For this review, take the finished solid that the model builds, in its own axes (mm). Coordinates: 2 decimals unless noted, no trailing zeros. Loops run counter-clockwise (first coordinate to the right, second up) from the corner with the lowest first, then second, coordinate; pieces in that order, holes last. Notation, with made-up numbers: M -18.5,31 L -5.5,31 A15 ccw -5.5,42 Z; hole C 49.25,-35 d1. An arc over 180 degrees is marked long. Use one line per item in the form item = value.
```python
from build123d import *

# Parameters (mm, degrees)
BOSS_EXTRUDE1_START = 63.5
BOSS_EXTRUDE1_DEPTH = 12.7
CAVITY1_START       = 63.5
CAVITY1_OUTLINE_R   = 12.7
CAVITY1_DEPTH       = 12.7


# Read off the part's stored shape, not the designer's step: Cavity1
with BuildPart() as part:
    # Sketch1 → Boss-Extrude1 (new body)
    with BuildSketch(Plane.XY.offset(BOSS_EXTRUDE1_START)):
        Polygon((2188.405431846, 757.059372145), (2594.805431846, 375.625791085), (2476.5, 375.625791085), (2476.5, 413.725791085), (2463.8, 413.725791085), (2463.8, 375.625791085), (2247.9, 375.625791085), (2247.9, 502.625791085), (2235.2, 502.625791085), (2235.2, 376.059372145), (2188.405431846, 376.059372145), align=None)
    extrude(amount=BOSS_EXTRUDE1_DEPTH)

    # Cavity1 outline → Cavity1 (cut)
    with BuildSketch(Plane.XY.offset(CAVITY1_START)):
        with Locations((2364.733137895, 514.21976629)):
            Circle(CAVITY1_OUTLINE_R)
    extrude(amount=CAVITY1_DEPTH, mode=Mode.SUBTRACT)


solid = part.part
```
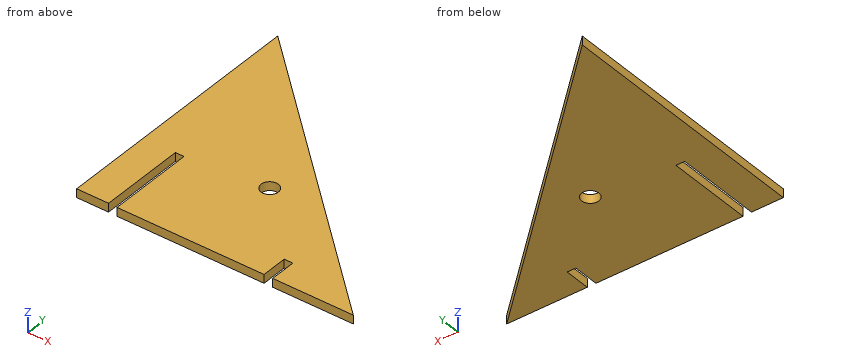
1. Wall thickness on line 1 along X through (y, z) = (465.5, 66.5); line 2 along X through (y, z) = (518, 72.5); line 3 along X through (y, z) = (601, 73): over which ranges is each line inside the solid? List them lowest first. Write a range as from..to.
Computed values:
line_1 = 2188.41..2235.2, 2247.9..2499.05
line_2 = 2188.41..2352.61, 2376.86..2443.11
line_3 = 2188.41..2354.68
2. Consider section A-A on x = 2359. Write out the cut boundary in (y, z), plus the area to 3 significant figures.
Computed values:
outline = M 375.63,63.5 L 502.89,63.5 L 502.89,76.2 L 375.63,76.2 Z; M 525.55,63.5 L 596.94,63.5 L 596.94,76.2 L 525.55,76.2 Z
area = 2,520 mm2
3. Consider section D-D on y = 674. Write out the cut boundary in (x, z).
Computed values:
outline = M 2188.41,63.5 L 2276.9,63.5 L 2276.9,76.2 L 2188.41,76.2 Z
4. For pin 1 Ø4 at (y, z) = (408.5, 69.5) entering from +X; pin 2 Ø1 at (x, z) = (2274, 68.5) entering from +Y; pin 3 Ø5 at (y, z) = (642.5, 67) entering from +X, all flat-tipped, find the tip position at first contact; note any pin that passes through.
Computed values:
pin_1 = 2561.91
pin_2 = 677.19
pin_3 = 2313.13
5. Consider section C-C on z = 68. Write out the cut boundary in (x, y).
Computed values:
outline = M 2188.41,376.06 L 2235.2,376.06 L 2235.2,502.63 L 2247.9,502.63 L 2247.9,375.63 L 2463.8,375.63 L 2463.8,413.73 L 2476.5,413.73 L 2476.5,375.63 L 2594.81,375.63 L 2188.41,757.06 Z; hole C 2364.73,514.22 d25.4
6. Consider section B-B on y = 473.5. Write out the cut boundary in (x, z), plus the area to 3 significant figures.
Computed values:
outline = M 2188.41,63.5 L 2235.2,63.5 L 2235.2,76.2 L 2188.41,76.2 Z; M 2247.9,63.5 L 2490.52,63.5 L 2490.52,76.2 L 2247.9,76.2 Z
area = 3,680 mm2
